```python
from build123d import *

# Parameters (mm, degrees)
SKETCH1_R           = 22.225
BOSS_EXTRUDE1_DEPTH = 6.35
SKETCH2_R           = 22.225
SKETCH2_R_2         = 19.05
BOSS_EXTRUDE2_DEPTH = 19.05
SKETCH3_R           = 19.05
SKETCH3_R_2         = 2.75
BOSS_EXTRUDE3_DEPTH = 3


with BuildPart() as part:
    # Sketch1 → Boss-Extrude1 (new body)
    with BuildSketch(Plane(origin=(0, 0, 0), x_dir=(1, 0, 0), z_dir=(0, 1, 0))):
        Circle(SKETCH1_R)
        Polygon((4.730817752, 7.253920553), (-3.9166706, 7.723968631), (-8.647488352, 0.470048077), (-4.730817752, -7.253920553), (3.9166706, -7.723968631), (8.647488352, -0.470048077), align=None, mode=Mode.SUBTRACT)
    extrude(amount=BOSS_EXTRUDE1_DEPTH)

    # Sketch2 → Boss-Extrude2 (add)
    with BuildSketch(Plane(origin=(0, 6.35, 0), x_dir=(1, 0, 0), z_dir=(0, 1, 0))):
        Circle(SKETCH2_R)
        Circle(SKETCH2_R_2, mode=Mode.SUBTRACT)
    extrude(amount=BOSS_EXTRUDE2_DEPTH)

    # Sketch3 → Boss-Extrude3 (add)
    with BuildSketch(Plane(origin=(0, 6.35, 0), x_dir=(1, 0, 0), z_dir=(0, 1, 0))):
        Circle(SKETCH3_R)
        Circle(SKETCH3_R_2, mode=Mode.SUBTRACT)
    extrude(amount=BOSS_EXTRUDE3_DEPTH)


solid = part.part
```
Can you work these out from the model? Positions are in its coordinate system, mm. A direction names the side the tool comes from. Coordinates: 2 decimals unless noted, no trailing zeros. Order: outer loops, then holes, each group sorted by start corner. A loop starts at its lowest first (then second) coordinate and runs counter-clockwise, first axis right, second up.
1. For faces 1 (the face through (4, 9.35, 0)), 2 (the face through (-6.717, 3.131, 3.338)), 3 (the face through (-0.596, 7.829, 2.685)), which set-ups out of +Z, -Z, +X, -X, +Y, -Y let a thin tool reach every point of the face, with its end or its side?
2. If we section it at A-A (y = 4.75): Please give me the cut outline in (x, z) (3 decimals).
3. If we section it at C-C (x = 0): Please give me the cut outline in (y, z) (3 decimals), then the cut area to 3 significant figures.
4. Thinking about a two-plate mould opening in Z: for faces 4 (the face through (0, 0, 10)), 5 (the face through (-6.249, 3.131, -4.148)), 6 (the face through (21.199, 12.522, -6.676)), which applies, +Z half, -Z half, draft (parallel to the pull), parting line (faces both ways), or undercut?
5. If we section it at B-B (z = 15.5): Please give me the cut outline in (x, y), then the cut area to 3 significant figures.
6. I'm going to push flat-ended pins straight in: pin 1 (4 mm diameter, centred on x = 8, z = 10, fed in from +Y); pin 2 (1 mm diameter, centred on x = 5.5, z = 7, fed in from -Y); pin 3 (1.5 mm diameter, centred on y = 17, z = -1, fed in from +X); pin 4 (3.5 mm diameter, centred on x = 0, z = 0, fed in from -Y) (1 decimal). Where does each tip first touch, or does it pass through?
7. If we section it at D-D (y = 11.5): Please give me the cut outline in (x, z) (3 decimals), then the cut area to 3 significant figures.
8. I need wall thicknesses on line 1 (X direction, y = 7.1, z = 0) (3 decimals); line 2 (X direction, y = 17.5, z = 0) (3 decimals). Which ranges of each line are inside material? Lowest first, please.
Entries:
1. face 1: +Y
1. face 2: -Y
1. face 3: +Y, -Y
2. outline: circle Ø44.45 at (0, 0); hole (-8.647, -0.47) - (-3.917, -7.724) - (4.731, -7.254) - (8.647, 0.47) - (3.917, 7.724) - (-4.731, 7.254) - close
3. outline: (0, -22.225) - (25.4, -22.225) - (25.4, -19.05) - (9.35, -19.05) - (9.35, -2.75) - (6.35, -2.75) - (6.35, -7.511) - (0, -7.511) - close; (0, 7.511) - (6.35, 7.511) - (6.35, 2.75) - (9.35, 2.75) - (9.35, 19.05) - (25.4, 19.05) - (25.4, 22.225) - (0, 22.225) - close
3. area: 406 mm2
4. face 4: draft
4. face 5: undercut
4. face 6: parting line
5. outline: (-15.93, 0) - (15.93, 0) - (15.93, 25.4) - (11.07, 25.4) - (11.07, 9.35) - (-11.07, 9.35) - (-11.07, 25.4) - (-15.93, 25.4) - close
5. area: 454 mm2
6. pin 1: stops at y = 9.35
6. pin 2: stops at y = 0
6. pin 3: stops at x = 22.22
6. pin 4: passes through
7. outline: circle Ø44.45 at (0, 0); hole circle Ø38.1 at (0, 0)
7. area: 412 mm2
8. line 1: x = -22.225 to -2.75, 2.75 to 22.225
8. line 2: x = -22.225 to -19.05, 19.05 to 22.225
